Autodesk Inventor part; units mm, degrees
ref_plane "YZ Plane" through (0, 0, 0) normal (1, 0, 0) x (0, 1, 0)
ref_plane "XZ Plane" through (0, 0, 0) normal (0, 1, 0) x (-1, 0, 0)
ref_plane "XY Plane" through (0, 0, 0) normal (0, 0, 1) x (1, 0, 0)
sketch "Sketch1" plane through (0, 0, 0) normal (1, 0, 0) x (0, 1, 0)
  line L0 (0, 36.5286) -> (0, -127.7004)
  line L1 (0, 36.5286) -> (-8, 36.5286)
  line L2 (-8, 36.5286) -> (-8, -127.7004)
  line L3 (-8, -127.7004) -> (-5.4683, -127.7004)
  line L4 (-5.4683, -127.7004) -> (-2.7019, -127.7004)
  line L5 (-2.7019, -127.7004) -> (0, -127.7004)
  line L6 (-8, 36.5286) -> (-10, 36.5286)
  line L7 (-10, 36.5286) -> (-12, 36.5286)
  line L8 (-12, 36.5286) -> (-12, -127.7004)
  line L9 (-12, -127.7004) -> (-8, -127.7004)
  point P0 (0, 0)
  dimension "d0" = 164.229
  dimension "d1" = 8
  dimension "d2" = 2
  dimension "d3" = 2
extrude "Extrusion1" add sketch "Sketch1" along normal blind 5 contours L0 L5 L4 L3 L2 L1
sketch "Sketch2" plane through (0, 0, 0) normal (-1, 0, 0) x (0, 0, 1)
  point P0 (0, 0)
extrude "Extrusion2" add sketch "Sketch1" along normal blind 50 contours L2 L9 L8 L7 L6
sketch "Sketch3" plane through (50, 0, 0) normal (1, 0, 0) x (0, 0, -1)
  line L0 (-36.5286, -12) -> (127.7004, -12)
  line L1 (-36.5286, 0) -> (-36.5286, -12)
  line L2 (-36.5286, -12) -> (-36.5286, 0)
  line L3 (127.7004, -12) -> (127.7004, 0)
  line L4 (-36.5286, 0) -> (127.7004, 0)
  line L5 (127.7004, 0) -> (127.7004, -12)
  line L6 (127.7004, -12) -> (-36.5286, -12)
  point P0 (0, 0)
  dimension "d8" = 12
extrude "Extrusion3" add sketch "Sketch3" along normal blind 5
properties part number "Flange" material "Aluminum 6061-AHC"
Design review of the part built by this model. Coordinates are the model's own, in mm. A direction names the side the tool comes from. Coordinates: 2 decimals unless noted, no trailing zeros. Order: outer loops, then holes, each group sorted by start corner. A loop starts at its lowest first (then second) coordinate and runs counter-clockwise, first axis right, second up.
Item 1: Take a section at B-B, the plane z = -40.5. Write out the cut boundary in (x, y), then the cut area to 3 significant figures.
Item 2: For faces 1 (the flat face through (27, -9, -127.7)), 2 (the flat face through (5, -4, -44)), list the 3-axis set-ups (+Z, -Z, +X, -X, +Y, -Y) from which the entire face can be reached by the end or side of a thin tool; tool diameter is ignored.
Item 3: For pin 1 Ø5 at (x, z) = (43, -107.5) entering from +Y, flat-tipped, find the tip position at first contact; note if it passes through.
Item 4: The part is to be moulded in two halves that separate along X. For faces 3 (the flat face through (27, -12, -44)), 4 (the flat face through (50, -4, -44)), 5 (the flat face through (55, -6, -44)), say which applies: pulls with the +X half, pulls with the -X half, needs draft (parallel to the pull), parting line crosses it, or undercut.
Item 5: For line 1 (X direction, y = -2.5, z = 25); line 2 (Y direction, x = 21, z = -30), list the stretches that pass through material, from the lowest coordinate up.
Item 6: Take a section at A-A, the plane y = -3.75. Write out the cut boundary in (x, z), then the cut area to 3 significant figures.
Item 7: Take a section at C-C, the plane x = 7.5. Write out the cut boundary in (y, z).
The answers:
1. outline: (0, -12) - (55, -12) - (55, 0) - (50, 0) - (50, -8) - (5, -8) - (5, 0) - (0, 0) - close
1. area: 300 mm2
2. face 1: -Z, +X, -X, +Y, -Y
2. face 2: +Z, -Z, +Y
3. pin 1: stops at y = -8
4. face 3: needs draft
4. face 4: undercut
4. face 5: pulls with the +X half
5. line 1: x = 0 to 5, 50 to 55
5. line 2: y = -12 to -8
6. outline: (0, -127.7) - (5, -127.7) - (5, 36.53) - (0, 36.53) - close; (50, -127.7) - (55, -127.7) - (55, 36.53) - (50, 36.53) - close
6. area: 1,640 mm2
7. outline: (-12, -127.7) - (-8, -127.7) - (-8, 36.53) - (-12, 36.53) - close
